Study the drawing (mm; zero at the part's minimum x, y, z) and answer. A direction names the side the tool comes from. Give positions to 0.01 mm unless a question says otherwise; leave off trailing zeros. Loops run counter-clockwise (first coordinate to the right, second up) from the corner with the lowest first, then second, coordinate; pieces in that order, holes last. Notation, with made-up numbers: M 56,56.25 L 89,56.25 A20 cw 89,84.25 Z; hole C 60.5,48 d1. An arc over 180 degrees is marked long. Use one line per item in the form item = value. Start each with the question number.
1. The part is cut by section C-C (x = 48). Write down the section's boundary in (y, z).
2. Each of these flat-tipped pins is pushed along its axis until it touches: pin 1 Ø5.5 at (x, y) = (48, 8.5) entering from +Z; pin 2 Ø2 at (x, y) = (11, 3) entering from -Z; pin 3 Ø4 at (x, y) = (7, 8.5) entering from -Z. Where does it stop, or does it pass through?
3. For the marked faces 4, 5 and 6, determine the directions among +Z, -Z, +X, -X, +Y, -Y from which every point of the face is accessible in a straight line to the end or side of a thin tool.
4. The mould has two halves that part along Y. Classify the marked faces 1, 2 and 3: released by +Y, released by -Y, zero draft, split by the parting line, or undercut.
5. The part is cut by section D-D (y = 5). Write down the section's boundary in (x, z) (1 decimal).
6. The part is cut by section B-B (z = 10). Write down the section's boundary in (x, y) (1 decimal), and give its area (3 significant figures).
7. Straight lines are drawn through the part: line 1 (X direction, y = 8.75, z = 26); line 2 (Y direction, x = 48, z = 24.7); line 3 (Z direction, x = 27.5, y = 8). For each, find the intervals that lie inside material, in ascending order. Write a range as from..to.
8. The part is cut by section A-A (y = 8.5). Write down the section's boundary in (x, z) (1 decimal), and give its area (3 significant figures).
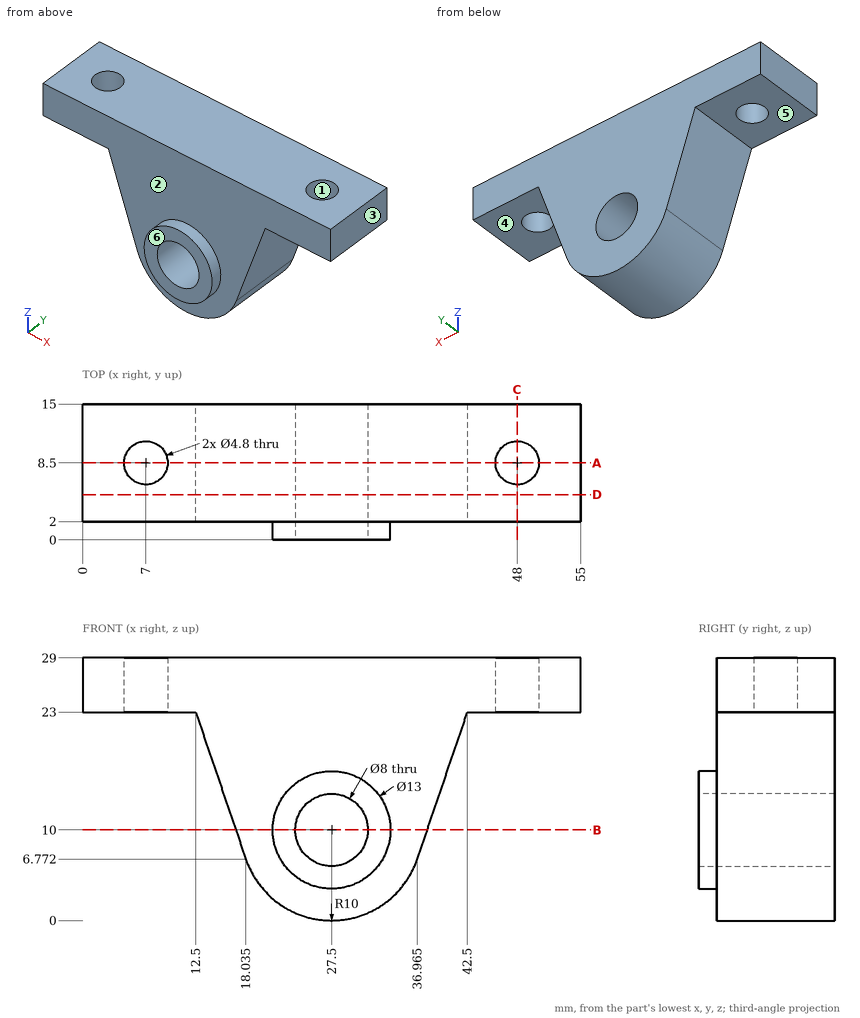
Derived:
q1.outline = M 2,23 L 6.1,23 L 6.1,29 L 2,29 Z; M 10.9,23 L 15,23 L 15,29 L 10.9,29 Z
q2.pin_1 = 29
q2.pin_2 = 23
q2.pin_3 = through
q3.face_4 = -Z, +X, +Y, -Y
q3.face_5 = -Z, -X, +Y, -Y
q3.face_6 = +Z, -Z, +X, -X, -Y
q4.face_1 = undercut
q4.face_2 = released by -Y
q4.face_3 = zero draft
q5.outline = M 0,23 L 12.5,23 L 18,6.8 A10 ccw 37,6.8 L 42.5,23 L 55,23 L 55,29 L 0,29 Z; hole C 27.5,10 d8
q6.outline = M 16.9,2 L 21,2 L 21,0 L 23.5,0 L 23.5,15 L 16.9,15 Z; M 31.5,0 L 34,0 L 34,2 L 38.1,2 L 38.1,15 L 31.5,15 Z
q6.area = 181 mm2
q7.line_1 = 0..4.61, 9.39..45.61, 50.39..55
q7.line_2 = 2..6.1, 10.9..15
q7.line_3 = 0..6, 14..29
q8.outline = M 0,23 L 4.6,23 L 4.6,29 L 0,29 Z; M 9.4,23 L 12.5,23 L 18,6.8 A10 ccw 37,6.8 L 42.5,23 L 45.6,23 L 45.6,29 L 9.4,29 Z; M 50.4,23 L 55,23 L 55,29 L 50.4,29 Z; hole C 27.5,10 d8
q8.area = 713 mm2
